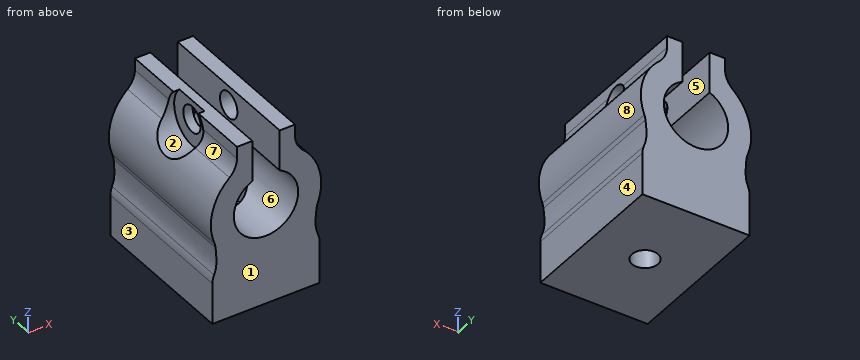
```python
from build123d import *

# Parameters (mm, degrees)
F1_DEPTH     = 20
F2_R         = 3.5
F2_R_2       = 1.7
F3_DEPTH     = 4
F4_DEPTH     = 25
F5_T1_DEPTH  = 20
F5_T6_DEPTH  = 12.1022846539
F5_S7_R      = 1.7
F5_T8_DEPTH  = 8
F5_T12_DEPTH = 12.1022846539
F5_S13_R     = 1.7
F5_T14_DEPTH = 8
F5_T18_DEPTH = 10.2630041323
F5_S19_R     = 3.5
F5_T20_DEPTH = 7
F5_T24_DEPTH = 10.2630041323
F5_S25_R     = 3.5
F5_T26_DEPTH = 7
F5_T27_DEPTH = 23.3663915102
F5_T29_DEPTH = 22.9020360067
F6_R         = 3.5
F6_R_2       = 1.7
F7_DEPTH     = 12
F8_DEPTH     = 12
F9_DEPTH     = 6


# Not quite as in the source:
# - a fillet or chamfer that OpenCascade refuses, or shapes differently, is made with other operations: its cross-section is extruded or revolved along the edge and cut away or added


with BuildPart() as f1:
    # F0 (on Front) → F1 (new body)
    with BuildSketch(Plane.XZ):
        with BuildLine():
            ThreePointArc((1.7894736842, 3.7997084011), (0, -4.2), (-1.7894736842, 3.7997084011))
            Line((-1.7894736842, 3.7997084011), (-1.7894736842, 9.1220820965))
            Line((-1.7894736842, 9.1220820965), (-3.7894736842, 9.1220820965))
            Line((-3.7894736842, 9.1220820965), (-3.7894736842, 6.1220820965))
            ThreePointArc((-3.7894736842, 6.1220820965), (-6.8557776995, 2.199616361), (-6.6439040907, -2.7746240166))
            add(Edge.make_bspline(
                [(-6.6356726702, -2.7942527112), (-6.6390399212, -2.7803089062), (-6.6413283577, -2.7774058988), (-6.6439040907, -2.7746240166)],
                knots=[0.9532514843, 0.9532514843, 0.9532514843, 0.9532514843, 1, 1, 1, 1], degree=3))
            add(Edge.make_bspline(
                [(-7, -7.2), (-6.7795680226, -6.7700727801), (-6.2785456929, -5.7974600377), (-6.5973790049, -2.9528269921), (-6.6356726702, -2.7942527112)],
                knots=[0, 0, 0, 0, 0.4216094964, 0.9532514843, 0.9532514843, 0.9532514843, 0.9532514843], degree=3))
            Line((-7, -7.2), (-7, -13.2))
            Line((-7, -13.2), (7, -13.2))
            Line((7, -13.2), (7, -7.2))
            add(Edge.make_bspline(
                [(7, -7.2), (6.7871491537, -6.6864508711), (6.3058923114, -5.5253136877), (6.5175995563, -3.7720698099), (6.6356726702, -2.7942527112)],
                knots=[0, 0, 0, 0, 0.4422811845, 1, 1, 1, 1], degree=3))
            ThreePointArc((6.6356726702, -2.7942527112), (6.8590214848, 2.1894803656), (3.7894736842, 6.1220820965))
            Line((3.7894736842, 6.1220820965), (3.7894736842, 9.1220820965))
            Line((3.7894736842, 9.1220820965), (1.7894736842, 9.1220820965))
            Line((1.7894736842, 9.1220820965), (1.7894736842, 3.7997084011))
        make_face()
        with BuildLine():
            add(Edge.make_bspline(
                [(-6.6356726702, -2.7942527112), (-6.6390399212, -2.7803089062), (-6.6413283577, -2.7774058988), (-6.6439040907, -2.7746240166)],
                knots=[0.9532514843, 0.9532514843, 0.9532514843, 0.9532514843, 1, 1, 1, 1], degree=3))
            ThreePointArc((-6.6439040907, -2.7746240166), (-6.6397956338, -2.7844414056), (-6.6356726702, -2.7942527112))
        make_face()
    extrude(amount=F1_DEPTH)

    # F2 (on face) → F3 (cut)
    with BuildSketch(Plane(origin=(-7, 0, 0), x_dir=(0, -1, 0), z_dir=(-1, 0, 0))):
        with Locations((10, 6.622)):
            Circle(F2_R)
        with Locations((10, 6.622)):
            Circle(F2_R_2, mode=Mode.SUBTRACT)
    extrude(amount=-F3_DEPTH, mode=Mode.SUBTRACT)

    # F2 (on face) → F4 (cut)
    with BuildSketch(Plane(origin=(-7, 0, 0), x_dir=(0, -1, 0), z_dir=(-1, 0, 0))):
        with Locations((10, 6.622)):
            Circle(F2_R_2)
    extrude(amount=-F4_DEPTH, mode=Mode.SUBTRACT)

    # F5: fillet of radius 3 on 8 edges, made by hand

    # F5_s2 → F5_t1 (join)
    with BuildSketch(Plane.XZ):
        with BuildLine():
            ThreePointArc((-6.5767127025, -3.2402461743), (-6.6395606645, -2.8691274316), (-6.7483493849, -2.5087886996))
            Line((-6.7483493849, -2.5087886996), (-6.466927581, -2.4041663985))
            ThreePointArc((-6.466927581, -2.4041663985), (-6.4145893512, -2.5416001874), (-6.3589651198, -2.6777323732))
            Line((-6.3589651198, -2.6777323732), (-6.343821894, -2.723774473))
            ThreePointArc((-6.343821894, -2.723774473), (-6.304537605, -2.9799785061), (-6.2781272304, -3.2087696206))
            Line((-6.2781272304, -3.2087696206), (-6.5767127025, -3.2402461743))
        make_face()
        with BuildLine():
            ThreePointArc((6.5887317904, -3.1834061265), (6.6509501418, -2.8334452349), (6.754091056, -2.4932898281))
            Line((6.754091056, -2.4932898281), (6.4724298111, -2.3893138658))
            ThreePointArc((6.4724298111, -2.3893138658), (6.4175024363, -2.534235691), (6.3589651198, -2.6777323732))
            Line((6.3589651198, -2.6777323732), (6.3375979172, -2.7582596669))
            ThreePointArc((6.3375979172, -2.7582596669), (6.3141276632, -2.9530960278), (6.290534619, -3.1484417941))
            Line((6.290534619, -3.1484417941), (6.5887317904, -3.1834061265))
        make_face()
    extrude(amount=F5_T1_DEPTH)


with BuildPart() as f5_tool4:
    # F5_s5 → F5_t6 (new body)
    with BuildSketch(Plane.XZ.offset(7.8977153461)):
        with BuildLine():
            ThreePointArc((4.792775332, 5.3724803189), (4.0514647707, 6.385428811), (3.7890736842, 7.6129290813))
            Line((3.7890736842, 7.6129290813), (3.4888336842, 7.6129290813))
            ThreePointArc((3.4888336842, 7.6129290813), (3.4892336842, 6.8675055889), (3.4892336842, 6.1220820965))
            Line((3.4892336842, 6.1220820965), (3.6314526316, 5.8667912731))
            ThreePointArc((3.6314526316, 5.8667912731), (4.1279416848, 5.5287236777), (4.5929054968, 5.1484354427))
            Line((4.5929054968, 5.1484354427), (4.792775332, 5.3724803189))
        make_face()
    extrude(amount=F5_T6_DEPTH)

    # F5_s7 → F5_t8 (cut, symmetric)
    with BuildSketch(Plane.YZ.offset(4.1)):
        with Locations((-10, 6.622)):
            Circle(F5_S7_R)
    extrude(amount=F5_T8_DEPTH, both=True, mode=Mode.SUBTRACT)


with BuildPart() as f1_1:
    add(f1.part)

    # F5_t3: union F5_tool4
    add(f5_tool4.part)


with BuildPart() as f5_tool10:
    # F5_s11 → F5_t12 (new body)
    with BuildSketch(Plane.XZ):
        with BuildLine():
            ThreePointArc((4.792775332, 5.3724803189), (4.0514647707, 6.385428811), (3.7890736842, 7.6129290813))
            Line((3.7890736842, 7.6129290813), (3.4888336842, 7.6129290813))
            ThreePointArc((3.4888336842, 7.6129290813), (3.4892336842, 6.8675055889), (3.4892336842, 6.1220820965))
            Line((3.4892336842, 6.1220820965), (3.6314526316, 5.8667912731))
            ThreePointArc((3.6314526316, 5.8667912731), (4.1279416848, 5.5287236777), (4.5929054968, 5.1484354427))
            Line((4.5929054968, 5.1484354427), (4.792775332, 5.3724803189))
        make_face()
    extrude(amount=F5_T12_DEPTH)

    # F5_s13 → F5_t14 (cut, symmetric)
    with BuildSketch(Plane.YZ.offset(4.1)):
        with Locations((-10, 6.622)):
            Circle(F5_S13_R)
    extrude(amount=F5_T14_DEPTH, both=True, mode=Mode.SUBTRACT)


with BuildPart() as f1_2:
    add(f1_1.part)

    # F5_t9: union F5_tool10
    add(f5_tool10.part)


with BuildPart() as f5_tool16:
    # F5_s17 → F5_t18 (new body)
    with BuildSketch(Plane.XZ):
        with BuildLine():
            ThreePointArc((-3.7890736842, 7.6129290813), (-4.0514647707, 6.385428811), (-4.792775332, 5.3724803189))
            Line((-4.792775332, 5.3724803189), (-4.5929054968, 5.1484354427))
            ThreePointArc((-4.5929054968, 5.1484354427), (-4.1279416848, 5.5287236777), (-3.6314526316, 5.8667912731))
            Line((-3.6314526316, 5.8667912731), (-3.4892336842, 6.1220820965))
            ThreePointArc((-3.4892336842, 6.1220820965), (-3.4892336842, 6.8675055889), (-3.4888336842, 7.6129290813))
            Line((-3.4888336842, 7.6129290813), (-3.7890736842, 7.6129290813))
        make_face()
    extrude(amount=F5_T18_DEPTH)

    # F5_s19 → F5_t20 (cut, symmetric)
    with BuildSketch(Plane.YZ.offset(-4.1)):
        with Locations((-10, 6.622)):
            Circle(F5_S19_R)
    extrude(amount=F5_T20_DEPTH, both=True, mode=Mode.SUBTRACT)


with BuildPart() as f1_3:
    add(f1_2.part)

    # F5_t15: union F5_tool16
    add(f5_tool16.part)


with BuildPart() as f5_tool22:
    # F5_s23 → F5_t24 (new body)
    with BuildSketch(Plane.XZ.offset(9.7369958677)):
        with BuildLine():
            ThreePointArc((-4.792775332, 5.3724803189), (-4.0514647707, 6.385428811), (-3.7890736842, 7.6129290813))
            Line((-3.7890736842, 7.6129290813), (-3.4888336842, 7.6129290813))
            ThreePointArc((-3.4888336842, 7.6129290813), (-3.4892336842, 6.8675055889), (-3.4892336842, 6.1220820965))
            Line((-3.4892336842, 6.1220820965), (-3.6314526316, 5.8667912731))
            ThreePointArc((-3.6314526316, 5.8667912731), (-4.1279416848, 5.5287236777), (-4.5929054968, 5.1484354427))
            Line((-4.5929054968, 5.1484354427), (-4.792775332, 5.3724803189))
        make_face()
    extrude(amount=F5_T24_DEPTH)

    # F5_s25 → F5_t26 (cut, symmetric)
    with BuildSketch(Plane.YZ.offset(-4.1)):
        with Locations((-10, 6.622)):
            Circle(F5_S25_R)
    extrude(amount=F5_T26_DEPTH, both=True, mode=Mode.SUBTRACT)


with BuildPart() as f1_4:
    add(f1_3.part)

    # F5_t21: union F5_tool22
    add(f5_tool22.part)

    # F5_s28 → F5_t27 (cut)
    with BuildSketch(Plane.XZ.offset(-1.6831957551)):
        with BuildLine():
            ThreePointArc((-7.0004, -7.8732781832), (-6.9416848839, -7.2824101234), (-6.7678360085, -6.7146521667))
            Line((-6.7678360085, -6.7146521667), (-7.0448196093, -6.5987895651))
            ThreePointArc((-7.0448196093, -6.5987895651), (-7.148871707, -6.8283644641), (-7.2671697753, -7.0630169034))
            Line((-7.2671697753, -7.0630169034), (-7.30024, -7.2))
            ThreePointArc((-7.30024, -7.2), (-7.30024, -7.5366390916), (-7.30064, -7.8732781832))
            Line((-7.30064, -7.8732781832), (-7.0004, -7.8732781832))
        make_face()
    extrude(amount=F5_T27_DEPTH, mode=Mode.SUBTRACT)

    # F5_s30 → F5_t29 (cut)
    with BuildSketch(Plane.XZ.offset(-1.4510180034)):
        with BuildLine():
            ThreePointArc((7.0004, -7.7804070635), (6.9510099307, -7.2380620544), (6.8044646756, -6.7135604089))
            Line((6.8044646756, -6.7135604089), (7.0851111432, -6.6068757434))
            ThreePointArc((7.0851111432, -6.6068757434), (7.178454263, -6.8447161783), (7.277360411, -7.0850423555))
            Line((7.277360411, -7.0850423555), (7.30024, -7.2))
            ThreePointArc((7.30024, -7.2), (7.30024, -7.4902035318), (7.30064, -7.7804070635))
            Line((7.30064, -7.7804070635), (7.0004, -7.7804070635))
        make_face()
    extrude(amount=F5_T29_DEPTH, mode=Mode.SUBTRACT)

    # F6 (on face) → F7 (cut)
    with BuildSketch(Plane(origin=(0, 0, -13.2), x_dir=(1, 0, 0), z_dir=(0, 0, -1))):
        with Locations((0, 10)):
            Circle(F6_R)
        with Locations((0, 10)):
            Circle(F6_R_2, mode=Mode.SUBTRACT)
    extrude(amount=-F7_DEPTH, mode=Mode.SUBTRACT)

    # F8 (cut): a face of the model
    f8_faces = [f1_4.faces().sort_by_distance(p)[0] for p in [
        (0, -10, -13.2),
    ]]
    extrude(f8_faces, amount=-F8_DEPTH, mode=Mode.SUBTRACT)

    # F6 (on face) → F9 (join)
    with BuildSketch(Plane(origin=(0, 0, -13.2), x_dir=(1, 0, 0), z_dir=(0, 0, -1))):
        with Locations((0, 10)):
            Circle(F6_R)
        with Locations((0, 10)):
            Circle(F6_R_2, mode=Mode.SUBTRACT)
    extrude(amount=-F9_DEPTH)


solid = f1_4.part
```
The model under review builds one solid part; all positions refer to its coordinate system, in mm. Face numbers are marked on the shaded views. A direction names the side the tool comes from. Round coordinates to 2 decimals unless told otherwise and drop trailing zeros. Loops run counter-clockwise (first coordinate to the right, second up) from the corner with the lowest first, then second, coordinate; pieces in that order, holes last. Notation, with made-up numbers: (-3, 40.25) -> (56, 40.25) arc R18 ccw to (56, 75.25) -> close; hole circle Ø5 at (19.25, 77). An arc over 180 degrees is marked (long way). Answer as a JSON object with one key per item and string values. Group by question number.
1) We need section B-B on z = 0. Write out the cut boundary in (x, y), then the cut area to 3 significant figures.
2) For the marked faces 1, 2, 3, 4 and 5, list the 3-axis set-ups (+Z, -Z, +X, -X, +Y, -Y) from which the entire face can be reached by the end or side of a thin tool; tool diameter is ignored.
3) For line 1 (Y direction, x = 0, z = -10.65); line 2 (X direction, y = -10, z = -11.35); line 3 (Z direction, x = 2.75, y = -11.5), list the stretches that pass through material, from the lowest coordinate up. Write a range as [from, to].
4) We need section D-D on z = 5.75. Write out the cut boundary in (x, y), then the cut area to 3 significant figures.
5) For pin 1 Ø1.8 at (y, z) = (-10, 7) entering from -X; pin 2 Ø2.5 at (y, z) = (-8.5, 6) entering from -X; pin 3 Ø1.6 at (y, z) = (-6.5, -9) entering from +X; pin 4 Ø1.6 at (y, z) = (-6, -12) entering from -X, all flat-tipped, find the tip position at first contact; note any pin that passes through.
6) Mouldability with a two-part tool opening along X and no side actions: class the marked faces 6, 7 and 8 as released by +X, released by -X, zero draft, split by the parting line, or undercut.
7) We need section A-A on x = 0. Write out the cut boundary in (y, z), then the cut area to 3 significant figures.
8) We need section C-C on x = -2.25. Write out the cut boundary in (y, z), then the cut area to 3 significant figures.
Result set:
{
 "1": {"outline": "(-7.2, -20) -> (-4.2, -20) -> (-4.2, 0) -> (-7.2, 0) -> close; (4.2, -20) -> (7.2, -20) -> (7.2, 0) -> (4.2, 0) -> close", "area": "120 mm²"},
 "2": {"face 1": "+Z, -Z, +X, -X, -Y", "face 2": "-X", "face 3": "-Z, -X, +Y, -Y", "face 4": "-Z, +X, +Y, -Y", "face 5": "+Z, +Y, -Y"},
 "3": {"line 1": "[-20, -11.7], [-8.3, 0]", "line 2": "[-7, -1.7], [1.7, 7]", "line 3": "[-13.2, -7.2], [3.17, 5.82], [7.42, 9.12]"},
 "4": {"outline": "(-4.44, -20) -> (-1.79, -20) -> (-1.79, -11.46) -> (-3, -11.46) -> (-3, -13.39) -> (-4.44, -13.39) -> close; (-4.44, -6.61) -> (-3, -6.61) -> (-3, -8.54) -> (-1.79, -8.54) -> (-1.79, 0) -> (-4.44, 0) -> close; (1.79, -20) -> (4.44, -20) -> (4.44, -11.46) -> (1.79, -11.46) -> close; (1.79, -8.54) -> (4.44, -8.54) -> (4.44, 0) -> (1.79, 0) -> close", "area": "84.9 mm²"},
 "5": {"pin 1": "through", "pin 2": "x = -3", "pin 3": "x = 7", "pin 4": "x = -7"},
 "6": {"face 6": "undercut", "face 7": "released by -X", "face 8": "released by +X"},
 "7": {"outline": "(-20, -13.2) -> (-11.7, -13.2) -> (-11.7, -7.2) -> (-13.5, -7.2) -> (-13.5, -4.2) -> (-20, -4.2) -> close; (-8.3, -13.2) -> (0, -13.2) -> (0, -4.2) -> (-6.5, -4.2) -> (-6.5, -7.2) -> (-8.3, -7.2) -> close", "area": "139 mm²"},
 "8": {"outline": "(-20, -13.2) -> (0, -13.2) -> (0, -3.55) -> (-7.32, -3.55) -> (-7.32, -7.2) -> (-12.68, -7.2) -> (-12.68, -3.55) -> (-20, -3.55) -> close; (-20, 3.55) -> (0, 3.55) -> (0, 9.12) -> (-20, 9.12) -> close; hole circle Ø3.4 at (-10, 6.62)", "area": "276 mm²"}
}
